```python
from build123d import *

# Parameters (mm, degrees)
F0_W         = 5.6
F0_H         = 4.5
F0_W_2       = 3.97
F0_H_2       = 2.5
F1_DEPTH     = 7.7
F2_W         = 5.6
F2_H         = 1.6
F3_DEPTH     = 4.5
F4_W         = 1.2
F4_H         = 2.5
F5_DEPTH     = 0.7
F8_DEPTH     = 6
F10_DEPTH    = 1
F12_DEPTH    = 2
F13_R        = 0.5
F14_T1_DEPTH = 4
F14_T3_DEPTH = 2.5


# Not quite as in the source:
# - a fillet or chamfer that OpenCascade refuses, or shapes differently, is made with other operations: its cross-section is extruded or revolved along the edge and cut away or added
# - a pattern or mirror of a feature is missing from the dataset's text; its kind, count and spacing are read off the source's solid


with BuildPart() as f1:
    # F0 (on Front) → F1 (new body)
    with BuildSketch(Plane.XZ):
        Rectangle(F0_W, F0_H)
        Rectangle(F0_W_2, F0_H_2, mode=Mode.SUBTRACT)
    extrude(amount=F1_DEPTH)

    # F2 (on face) → F3 (join)
    with BuildSketch(Plane(origin=(0, 0, -2.25), x_dir=(1, 0, 0), z_dir=(0, 0, -1))):
        with Locations((0, 5.5)):
            Rectangle(F2_W, F2_H)
    extrude(amount=F3_DEPTH)

    # F4 (on face) → F5 (join)
    with BuildSketch(Plane.YZ.offset(-1.985)):
        with Locations((-7.1, 0)):
            Rectangle(F4_W, F4_H)
    f5 = extrude(amount=F5_DEPTH)

    # F5_copies: F5 across plane
    add(f5.mirror(Plane(origin=(0, 0, 0), x_dir=(0, 0, 1), z_dir=(1, 0, 0))))

    # F7 (on face) → F8 (join)
    with BuildSketch(Plane.YZ.offset(2.8)):
        Polygon((0, 2.25), (-7.7, 2.25), (-7.7, -2.25), (-6.3, -2.25), (-4.7, -2.25), (0, -2.25), align=None)
    extrude(amount=F8_DEPTH)

    # F9 (on face) → F10 (cut)
    with BuildSketch(Plane.XY.offset(2.25)):
        with BuildLine():
            ThreePointArc((-1.0984344714, -5.5712931935), (-0.0293434956, -6.7295678482), (1.1, -5.6299593))
            ThreePointArc((1.1, -5.6299593), (1.0996085482, -5.6006158044), (1.0984344714, -5.5712931935))
            ThreePointArc((1.0984344714, -5.5712931935), (0.7567916764, -4.8316696542), (0, -4.5299593))
            ThreePointArc((0, -4.5299593), (-0.7567916764, -4.8316696542), (-1.0984344714, -5.5712931935))
        make_face()
        with BuildLine():
            ThreePointArc((1.0984344714, -5.5712931935), (1.0996085482, -5.6006158044), (1.1, -5.6299593))
            ThreePointArc((1.1, -5.6299593), (-0.0293434956, -6.7295678482), (-1.0984344714, -5.5712931935))
            Line((-1.0984344714, -5.5712931935), (-1.35, -7.7))
            Line((-1.35, -7.7), (1.35, -7.7))
            Line((1.35, -7.7), (1.0984344714, -5.5712931935))
        make_face()
    extrude(amount=-F10_DEPTH, mode=Mode.SUBTRACT)

    # F11 (on face) → F12 (join)
    with BuildSketch(Plane(origin=(-2.8, 0, 0), x_dir=(0, -1, 0), z_dir=(-1, 0, 0))):
        Polygon((7.7, -2.25), (7.7, 2.25), (0, 2.25), (0, -2.25), (4.7, -2.25), (6.3, -2.25), align=None)
    extrude(amount=F12_DEPTH)

    # F13
    f13_edges = [f1.edges().sort_by_distance(p)[0] for p in [
        (8.8, -3.85, -2.25),
        (8.8, -3.85, 2.25),
        (2.8, -5.5, -6.75),
        (-4.8, -3.85, 2.25),
        (-4.8, -3.85, -2.25),
        (-2.8, -5.5, -6.75),
    ]]
    fillet(f13_edges, radius=F13_R)

    # F14: fillet of radius 0.25 on 4 edges, made by hand

    # F14_s2 → F14_t1 (cut)
    with BuildSketch(Plane.XY.offset(-1.25)):
        with BuildLine():
            ThreePointArc((-1.535, -7.7), (-1.3582233047, -7.6267766953), (-1.285, -7.45))
            Line((-1.285, -7.45), (-1.28, -7.45))
            Line((-1.28, -7.45), (-1.28, -7.705))
            Line((-1.28, -7.705), (-1.535, -7.705))
            Line((-1.535, -7.705), (-1.535, -7.7))
        make_face()
        with BuildLine():
            ThreePointArc((1.535, -7.7), (1.3582233047, -7.6267766953), (1.285, -7.45))
            Line((1.285, -7.45), (1.28, -7.45))
            Line((1.28, -7.45), (1.28, -7.705))
            Line((1.28, -7.705), (1.535, -7.705))
            Line((1.535, -7.705), (1.535, -7.7))
        make_face()
    extrude(amount=F14_T1_DEPTH, mode=Mode.SUBTRACT)

    # F14_s4 → F14_t3 (cut)
    with BuildSketch(Plane.XY.offset(-1.25)):
        with BuildLine():
            ThreePointArc((-1.285, -6.75), (-1.3582233047, -6.5732233047), (-1.535, -6.5))
            Line((-1.535, -6.5), (-1.535, -6.495))
            Line((-1.535, -6.495), (-1.28, -6.495))
            Line((-1.28, -6.495), (-1.28, -6.75))
            Line((-1.28, -6.75), (-1.285, -6.75))
        make_face()
        with BuildLine():
            ThreePointArc((1.285, -6.75), (1.3582233047, -6.5732233047), (1.535, -6.5))
            Line((1.535, -6.5), (1.535, -6.495))
            Line((1.535, -6.495), (1.28, -6.495))
            Line((1.28, -6.495), (1.28, -6.75))
            Line((1.28, -6.75), (1.285, -6.75))
        make_face()
    extrude(amount=F14_T3_DEPTH, mode=Mode.SUBTRACT)


solid = f1.part
```
The listing builds one solid part. Answer for the finished solid, in the listing's coordinates (mm). A direction names the side the tool comes from. Coordinates: 2 decimals unless noted, no trailing zeros. Loops run counter-clockwise (first coordinate to the right, second up) from the corner with the lowest first, then second, coordinate; pieces in that order, holes last. Notation, with made-up numbers: M 78.25,56 L 95.25,56 A20 cw 95.25,80 Z; hole C -23.75,-30.5 d4. An arc over 180 degrees is marked long. Answer as CSV lines item,"result". Start each with the question number.
(1) The part is cut by section D-D (z = -3). Give the vertices of the cut face in (x, y), and give its area (3 significant figures).
(2) The part is cut by section A-A (z = -0.25). Give the vertices of the cut face in (x, y) (3 decimals), and give its area (3 significant figures).
(3) Given pin 1 (1.8 mm diameter, centred on y = -5.5, z = -3.5, fed in from +X); pin 2 (1.8 mm diameter, centred on y = -5.5, z = -4.5, fed in from -X); pin 3 (1 mm diameter, centred on y = -2, z = -3, fed in from -X); pin 4 (1.3 mm diameter, centred on x = 1.5, z = -5, fed in from -Y), each flat-ended and moving along its own axis, determine where each tip first touches the part or whether it passes through.
(4) For faces 4 (the flat face through (0, -6.3, -4)), 5 (the flat face through (2.8, -5, -4)), 6 (the flat face through (1.22, -6.6, 1.76)), 7 (the flat face through (-2.8, -5, -4)), determine the directions among +Z, -Z, +X, -X, +Y, -Y from which every point of the face is accessible in a straight line to the end or side of a thin tool.
(5) The part is cut by section B-B (y = -4.25). Give the vertices of the cut face in (x, z) (3 decimals).
(6) Find the intervals of material crossed by L1, parallel to X at y = -3.5, z = 1 (3 decimals); L2, parallel to Z at x = 6.5, y = -6.5; L3, parallel to Z at x = 0.75, y = -0.5, in increasing order. Write a range as [from, to].
(7) The mould has two halves that part along X. Classify faces 1 (the flat face through (-4.8, -4, 0)), 2 (the flat face through (2, -7.7, 0)), 3 (the flat face through (1.985, -3, 0)): pulls with the +X half, pulls with the -X half, needs draft (parallel to the pull), parting line crosses it, or undercut.
(8) The part is cut by section C-C (x = 0.75). Give the vertices of the cut face in (y, z).
Determined:
1,outline,"M -2.8,-6.3 L 2.8,-6.3 L 2.8,-4.7 L -2.8,-4.7 Z"
1,area,"8.96 mm2"
2,outline,"M -4.8,-7.7 L -1.535,-7.7 A0.25 ccw -1.285,-7.45 L -1.285,-6.75 A0.25 ccw -1.535,-6.5 L -1.985,-6.5 L -1.985,0 L -4.8,0 Z; M 1.285,-7.45 A0.25 ccw 1.535,-7.7 L 8.8,-7.7 L 8.8,0 L 1.985,0 L 1.985,-6.5 L 1.535,-6.5 A0.25 ccw 1.285,-6.75 Z"
2,area,"75.8 mm2"
3,pin 1,"x = 2.8"
3,pin 2,"x = -2.8"
3,pin 3,"through"
3,pin 4,"y = -6.3"
4,face 4,"-Z, +X, -X, -Y"
4,face 5,"-Z, +X, +Y, -Y"
4,face 6,"+Z, -Y"
4,face 7,"-Z, -X, +Y, -Y"
5,outline,"M -4.8,-1.75 A0.5 ccw -4.3,-2.25 L 8.3,-2.25 A0.5 ccw 8.8,-1.75 L 8.8,1.75 A0.5 ccw 8.3,2.25 L -4.3,2.25 A0.5 ccw -4.8,1.75 Z; hole M -1.985,-1.25 L 1.985,-1.25 L 1.985,1.25 L -1.985,1.25 Z"
6,L1,"[-4.8, -1.985], [1.985, 8.8]"
6,L2,"[-2.25, 2.25]"
6,L3,"[-2.25, -1.25], [1.25, 2.25]"
7,face 1,"pulls with the -X half"
7,face 2,"needs draft"
7,face 3,"undercut"
8,outline,"M -7.7,-2.25 L -6.3,-2.25 L -6.3,-6.75 L -4.7,-6.75 L -4.7,-2.25 L 0,-2.25 L 0,-1.25 L -7.7,-1.25 Z; M -4.83,1.25 L 0,1.25 L 0,2.25 L -4.83,2.25 Z"
